Check sheet for the modelled part. Datum: model origin and axes. Units: mm. A direction names the side the tool comes from. Round coordinates to 2 decimals unless told otherwise and drop trailing zeros. Write each loop counter-clockwise with the first axis right and the second up, starting at its lowest first coordinate (ties: lowest second). Pieces come first, ordered by that corner, then holes. Notation, with made-up numbers: M -13.75,26 L 45.25,26 A17 ccw 45.25,45 Z; hole C 84.5,-25.5 d11. An arc over 180 degrees is marked long. Answer in a Markdown table with one row per item.
```python
from build123d import *

# Parameters (mm, degrees)
SKETCH1_W           = 50
SKETCH1_H           = 700
BOSS_EXTRUDE1_DEPTH = 50
SKETCH2_W           = 45
SKETCH2_H           = 45
CUT_EXTRUDE1_DEPTH  = 704.562363974
CUT_EXTRUDE2_DEPTH  = 704.562363974
CHAMFER1_SIZE       = 5


with BuildPart() as part:
    # Sketch1 → Boss-Extrude1 (new body)
    with BuildSketch(Plane.XY):
        with Locations((25, 350)):
            Rectangle(SKETCH1_W, SKETCH1_H)
    extrude(amount=BOSS_EXTRUDE1_DEPTH)

    # Sketch2 → Cut-Extrude1 (cut, through all)
    with BuildSketch(Plane(origin=(0, 700, 0), x_dir=(1, 0, 0), z_dir=(0, 1, 0))):
        with Locations((25, -25)):
            Rectangle(SKETCH2_W, SKETCH2_H)
    extrude(amount=-CUT_EXTRUDE1_DEPTH, mode=Mode.SUBTRACT)

    # Sketch3 → Cut-Extrude2 (cut, through all)
    with BuildSketch(Plane.ZY):
        Polygon((0, 700), (50, 700), (50, 656.25), align=None)
        Polygon((0, 0), (50, 0), (50, 43.75), align=None)
    extrude(amount=-CUT_EXTRUDE2_DEPTH, mode=Mode.SUBTRACT)

    # Chamfer1
    chamfer1_edges = [part.edges().sort_by_distance(p)[0] for p in [
        (0, 350, 50),
        (50, 350, 50),
        (0, 350, 0),
        (50, 350, 0),
    ]]
    chamfer(chamfer1_edges, length=CHAMFER1_SIZE - 0.0001)  # a hair under: the kernel refuses the full size


solid = part.part
```
1. Section check B-B, the plane z = 28. Record the cut outline in (x, y), and give its area (4 significant figures).
Found:
| item | result |
|---|---|
| outline | M 0,24.5 L 2.5,24.5 L 2.5,675.5 L 0,675.5 Z; M 47.5,24.5 L 50,24.5 L 50,675.5 L 47.5,675.5 Z |
| area | 3,255 mm2 |
2. Scan lines: L1, parallel to X at y = 115.5, z = 34.5; L2, parallel to Z at x = 21.5, y = 670. Record each from-to range of solid material in increasing order.
Found:
| item | result |
|---|---|
| L1 | x = 0 to 2.5, 47.5 to 50 |
| L2 | z = 0 to 2.5 |
3. Access from +Z, -Z, +X, -X, +Y, -Y to the whole of each face (thin tool, end or side, straight path). Record for faces 1 (the face through (25, 354, 50)), 2 (the face through (47.5, 355, 25)).
Found:
| item | result |
|---|---|
| face 1 | +Z, +X, -X, +Y, -Y |
| face 2 | +Y, -Y |
4. Draft check along X on faces 3 (the face through (0.81, 678.02, 25.12)), 4 (the face through (2.5, 355, 25)), 5 (the face through (50, 345, 25)). Enter one of: +X half, -X half, draft (parallel to the pull), parting line (faces both ways), or undercut.
Found:
| item | result |
|---|---|
| face 3 | draft |
| face 4 | undercut |
| face 5 | +X half |
5. Go/stop test with a flat-tipped pin: pin 1 (8 mm diameter, centred on x = 44.5, z = 30, fed in from +Y). Record where the tip stops, or that it passes through.
Found:
| item | result |
|---|---|
| pin 1 | stops at y = 676.07 |
6. Section check C-C, the plane y = 123. Record the cut outline in (x, z).
Found:
| item | result |
|---|---|
| outline | M 0,5 L 5,0 L 45,0 L 50,5 L 50,45 L 45,50 L 5,50 L 0,45 Z; hole M 2.5,2.5 L 47.5,2.5 L 47.5,47.5 L 2.5,47.5 Z |
7. Section check A-A, the plane x = 16.5. Record the cut outline in (y, z).
Found:
| item | result |
|---|---|
| outline | M 0,0 L 700,0 L 697.81,2.5 L 2.19,2.5 Z; M 41.56,47.5 L 658.44,47.5 L 656.25,50 L 43.75,50 Z |
